Input: dimensioned drawing with shaded views. Units: mm. Origin: part minimum x, y, z. A direction names the side the tool comes from. Give positions to 0.01 mm unless a question says otherwise; leave off trailing zeros. Loops run counter-clockwise (first coordinate to the right, second up) from the corner with the lowest first, then second, coordinate; pieces in that order, holes last. Notation, with made-up numbers: (-25.75, 6.25) -> (19.25, 6.25) arc R21 cw to (19.25, 26.25) -> close; hole circle Ø11 at (29, -29). An arc over 180 degrees is marked (long way). Answer in a Markdown table with one row per item. Add a question column.
1) Section query A-A (x = 18). Return the cut outline in (y, z).
2) Section query C-C (y = 18.5). Return the cut outline in (x, z).
3) Section query B-B (z = 5). Return the cut outline in (x, y).
4) Line query: line 1 (Z direction, x = 13.5, y = 9.5); line 2 (Y direction, x = 14, z = 25.5); line 3 (X direction, y = 12, z = 2.5). Output: solid intervals per line, ascending. Write a range as from..to.
5) Access query for the marked faces 4 and 5. Directions: +Z, -Z, +X, -X, +Y, -Y. A direction counts if a zero-diameter tool reaches every point of the face in a straight line with its end or side. Return the directions, or none.
6) Draft query along Y for the marked faces 1, 2 and 3. Return one class per face: +Y half, -Y half, draft (parallel to the pull), parting line (faces both ways), or undercut.
7) First-contact query: P1, Ø2, axis at y = 14, z = 1.5, coming from the -X side; P2, Ø10, axis at y = 14.5, z = 14, coming from the -X side; P3, Ø2, axis at x = 4, y = 7, coming from the -Z side. Flat tips, straight axial feed; report the tip coordinate or a pass-through.
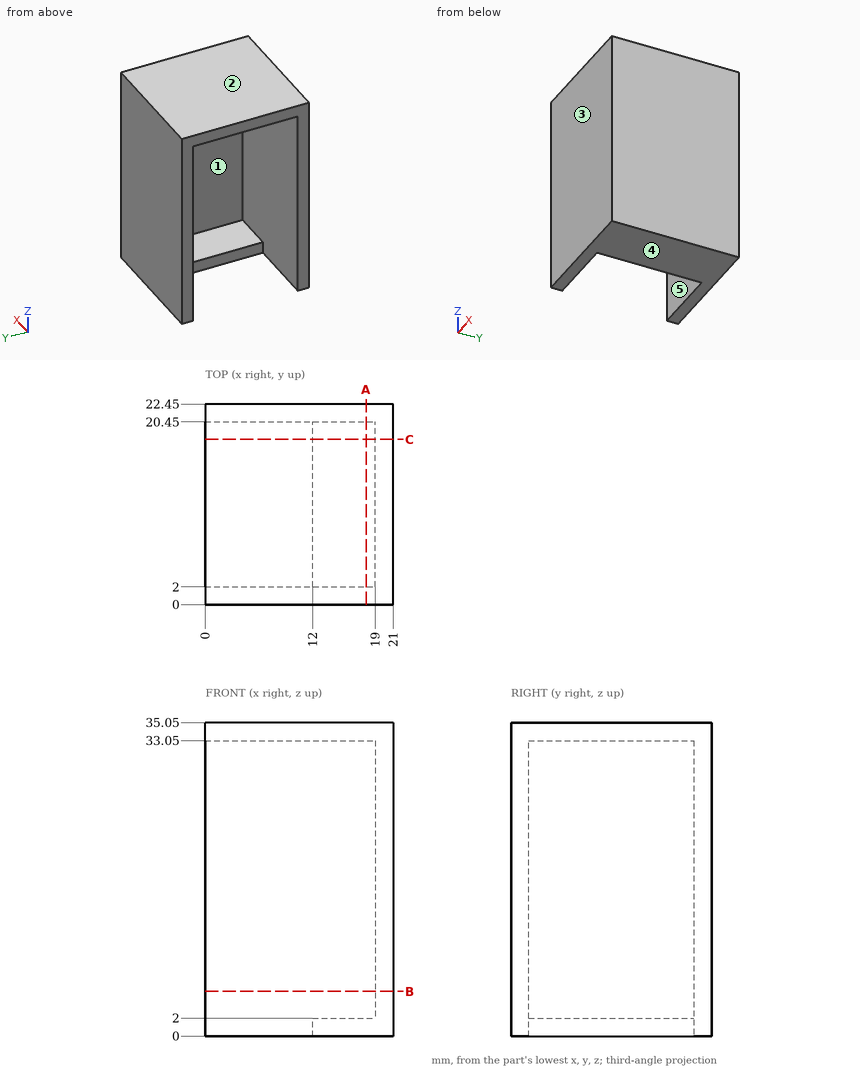
Evaluation:
| question | item | result |
|---|---|---|
| 1 | outline | (0, 0) -> (22.45, 0) -> (22.45, 35.05) -> (0, 35.05) -> close; hole (2, 2) -> (20.45, 2) -> (20.45, 33.05) -> (2, 33.05) -> close |
| 2 | outline | (0, 33.05) -> (19, 33.05) -> (19, 2) -> (12, 2) -> (12, 0) -> (21, 0) -> (21, 35.05) -> (0, 35.05) -> close |
| 3 | outline | (0, 0) -> (21, 0) -> (21, 22.45) -> (0, 22.45) -> (0, 20.45) -> (19, 20.45) -> (19, 2) -> (0, 2) -> close |
| 4 | line 1 | 0..2, 33.05..35.05 |
| 4 | line 2 | 0..2, 20.45..22.45 |
| 4 | line 3 | 19..21 |
| 5 | face 4 | -Z, +X, -X, +Y, -Y |
| 5 | face 5 | -X |
| 6 | face 1 | undercut |
| 6 | face 2 | draft |
| 6 | face 3 | -Y half |
| 7 | P1 | x = 12 |
| 7 | P2 | x = 19 |
| 7 | P3 | z = 33.05 |
